For this review, take the finished solid that the model builds, in its own axes (mm). A direction names the side the tool comes from. Give positions to 0.01 mm unless a question says otherwise; leave off trailing zeros. Loops run counter-clockwise (first coordinate to the right, second up) from the corner with the lowest first, then second, coordinate; pieces in that order, holes last. Notation, with made-up numbers: (36.25, -9) -> (54.25, -9) arc R30 ccw to (54.25, 23) -> close; hole circle Ø2 at (69, 33.25). An arc over 180 degrees is marked (long way). Answer as CSV lines item,"result". Start each with the question number.
Item 1: Machinability: for faces 1 (the face through (480, -550, 6)), 2 (the face through (480, -94, 6)), 3 (the face through (-20, -20, 6)), which of the approach directions +Z, -Z, +X, -X, +Y, -Y give a long, thin tool a straight path to every point of the face, cutting with its end or side? Answer none if there is none.
Item 2: The part is to be moulded in two halves that separate along X. For faces 4 (the face through (275, -86, 6)), 5 (the face through (0, -550, 6)), 6 (the face through (520, -276, 6)), 7 (the face through (243, -560, 6)), say which applies: +X half, -X half, draft (parallel to the pull), parting line (faces both ways), or undercut.
Item 3: Clearance check with flat-ended pins moving along their axes: P1, Ø6, axis at x = 505, z = 4, coming from the -Y side; P2, Ø3.5, axis at x = 497, z = 7.5, coming from the +Y side; P3, Ø4, axis at x = 312, y = -347, coming from the -Z side; P4, Ø6, axis at y = -5.5, z = 4, coming from the -X side. State where each tip first meets the part, or that it passes through.
Item 4: For L1, parallel to X at y = -33, z = 6.5; L2, parallel to Y at x = 464.5, z = 6.75; L3, parallel to Y at x = -3, z = 3.5, list the stretches that pass through material, from the lowest coordinate up. Write a range as from..to.
Item 5: Add section B-B on x = 317. State the section outline as (y, z) points.
Item 6: Add section A-A on z = 9.25. State the section outline as (x, y) points.
```python
from build123d import *

# Parameters (mm, degrees)
EXTRUDE_1_DEPTH     = 12
SKETCH_3_W          = 205
SKETCH_3_H          = 170
CUT_EXTRUDE_2_DEPTH = 12
SKETCH_4_W          = 12
SKETCH_4_H          = 150
EXTRUDE_2_DEPTH     = 2
SKETCH_5_W          = 2
SKETCH_5_H          = 12
CUT_EXTRUDE_3_DEPTH = 150


with BuildPart() as part:
    # ｽｹｯﾁ1 → ﾎﾞｽ - 押し出し1 (new body)
    with BuildSketch(Plane.XY):
        Polygon((0, 0), (480, 0), (480, -20), (520, -20), (520, -540), (480, -540), (480, -560), (0, -560), (0, -540), (-40, -540), (-40, -20), (0, -20), align=None)
    extrude(amount=EXTRUDE_1_DEPTH)

    # ｽｹｯﾁ3 → ｶｯﾄ - 押し出し2 (cut)
    with BuildSketch(Plane.XY.offset(12)):
        with Locations((377.5, -85)):
            Rectangle(SKETCH_3_W, SKETCH_3_H)
    extrude(amount=-CUT_EXTRUDE_2_DEPTH, mode=Mode.SUBTRACT)

    # ｽｹｯﾁ4 → ﾎﾞｽ - 押し出し2 (add)
    with BuildSketch(Plane.ZY.offset(-480)):
        with Locations((6, -95)):
            Rectangle(SKETCH_4_W, SKETCH_4_H)
    extrude(amount=EXTRUDE_2_DEPTH)

    # ｽｹｯﾁ5 → ｶｯﾄ - 押し出し3 (cut)
    with BuildSketch(Plane(origin=(0, -20, 0), x_dir=(1, 0, 0), z_dir=(0, 1, 0))):
        with Locations((479, -6)):
            Rectangle(SKETCH_5_W, SKETCH_5_H)
    extrude(amount=-CUT_EXTRUDE_3_DEPTH, mode=Mode.SUBTRACT)


solid = part.part
```
Computed values:
1,face 1,"+Z, -Z, +X, -Y"
1,face 2,"+Z, -Z, +Y"
1,face 3,"+Z, -Z, -X, +Y"
2,face 4,"undercut"
2,face 5,"-X half"
2,face 6,"+X half"
2,face 7,"draft"
3,P1,"y = -540"
3,P2,"y = -20"
3,P3,"z = 0"
3,P4,"x = 0"
4,L1,"-40..275, 480..520"
4,L2,"-560..-170"
4,L3,"-540..-20"
5,outline,"(-560, 0) -> (-170, 0) -> (-170, 12) -> (-560, 12) -> close"
6,outline,"(-40, -540) -> (0, -540) -> (0, -560) -> (480, -560) -> (480, -540) -> (520, -540) -> (520, -20) -> (480, -20) -> (480, -170) -> (275, -170) -> (275, 0) -> (0, 0) -> (0, -20) -> (-40, -20) -> close"
